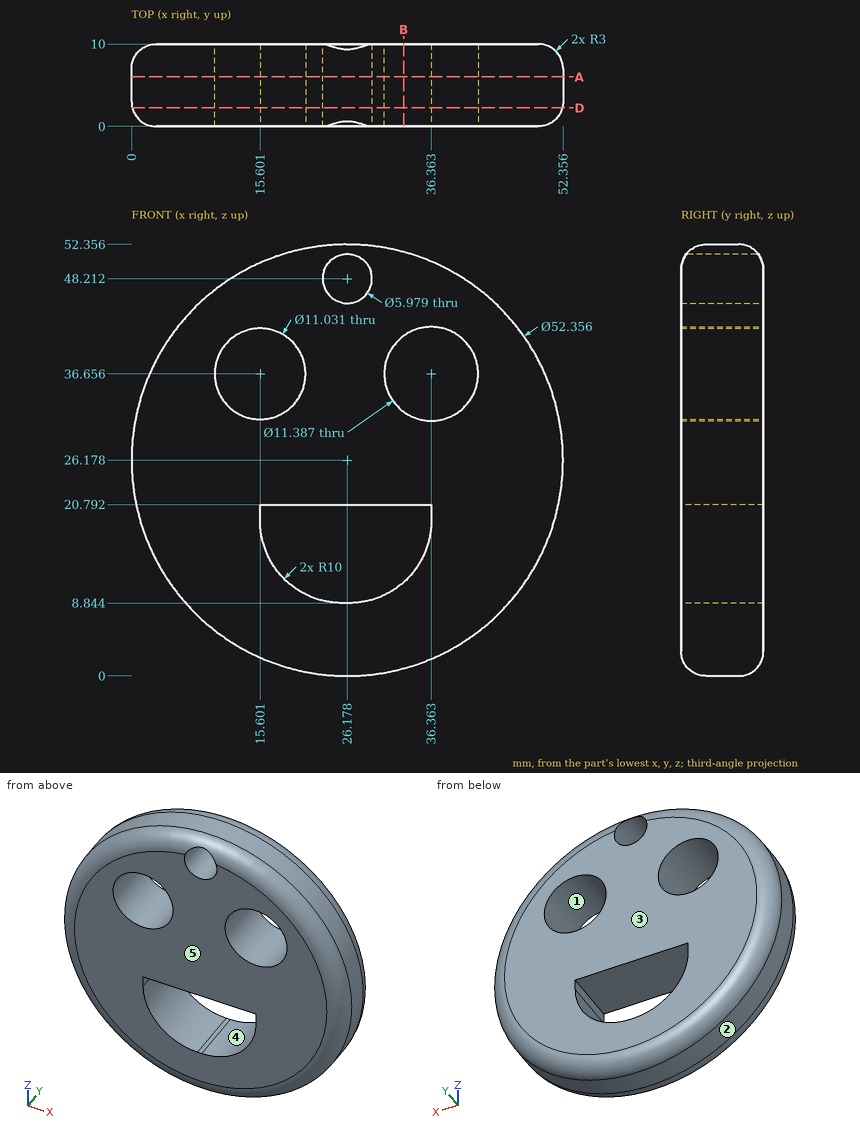
For this review, use the dimensioned drawing (mm, ordinates from the lowest corner) and the shaded views. A direction names the side the tool comes from. Round coordinates to 2 decimals unless told otherwise and drop trailing zeros. Loops run counter-clockwise (first coordinate to the right, second up) from the corner with the lowest first, then second, coordinate; pieces in that order, holes last. Notation, with made-up numbers: M 22.25,2.5 L 71.25,2.5 A7 cw 71.25,9.5 Z; hole C -39,25 d8. An arc over 180 degrees is marked long. Answer as CSV lines item,"result".
1. We need section B-B (x = 33). Count the separate pieces of the cut face and the enclosed holes in it, plus the area to 3 significant figures.
Outcome:
separate pieces,"3"
enclosed holes,"0"
area,"311 mm2"
2. For the marked faces 4 and 5, list the 3-axis set-ups (+Z, -Z, +X, -X, +Y, -Y) from which the entire face can be reached by the end or side of a thin tool; tool diameter is ignored.
Outcome:
face 4,"+Y, -Y"
face 5,"+Z, -Z, +X, -X, -Y"
3. Insertion check: pin 1 Ø1 at (y, z) = (8, 44.5) entering from -X; pin 2 Ø0.6 at (y, z) = (3.5, 20) entering from -X; pin 3 Ø10 at (x, z) = (15.6, 36.66) entering from -Y; pin 4 Ø1.5 at (y, z) = (8.5, 45) entering from -X. Each pin has a flat end and moves straight along its axis. Give the tip position at first contact, or say it passes through.
Outcome:
pin 1,"stops at x = 7.19"
pin 2,"stops at x = 0.67"
pin 3,"passes through"
pin 4,"stops at x = 7.64"
4. We need section A-A (y = 6). Give the boundary of the cut face in (x, z) (1 decimal), plus the area to 3 significant figures.
Outcome:
outline,"C 26.2,26.2 d52.4; hole C 15.6,36.7 d11; hole M 15.6,18.8 A10 ccw 25.6,8.8 L 26.4,8.8 A10 ccw 36.4,18.8 L 36.4,20.8 L 15.6,20.8 Z; hole C 26.2,48.2 d6; hole C 36.4,36.7 d11.4"
area,"1,720 mm2"
5. To check wall thickness, follow L1, parallel to X at y = 9, z = 41 (1 decimal); L2, parallel to Z at x = 19, y = 1.25 (1 decimal); L3, parallel to Z at x = 34, y = 6.25 (1 decimal). State the ranges of each line that lie inside material, in increasing order. Write a range as [from, to].
Outcome:
L1,"x = [5.5, 12.2], [19, 32.7], [40, 46.8]"
L2,"z = [1.6, 11.3], [20.8, 32.3], [41, 50.8]"
L3,"z = [1.2, 12.4], [20.8, 31.5], [41.8, 51.2]"
6. Draft analysis for pull direction Z (two halves, no side actions). For the marked faces 1, 2 and 3, state which applies: pulls with the +Z half, pulls with the -Z half, needs draft (parallel to the pull), parting line crosses it, or undercut.
Outcome:
face 1,"undercut"
face 2,"parting line crosses it"
face 3,"needs draft"
7. We need section D-D (y = 2.25). Give the boundary of the cut face in (x, z) (1 decimal).
Outcome:
outline,"C 26.2,26.2 d52.2; hole C 15.6,36.7 d11; hole M 15.6,18.8 A10 ccw 25.6,8.8 L 26.4,8.8 A10 ccw 36.4,18.8 L 36.4,20.8 L 15.6,20.8 Z; hole C 26.2,48.2 d6; hole C 36.4,36.7 d11.4"
